```python
from build123d import *

# Parameters (mm, degrees)
SKETCH001_W  = 448.31
SKETCH001_H  = 304.8
PAD_DEPTH    = 4.318
POCKET_DEPTH = 1088.576426


with BuildPart() as part:
    # Sketch001 → Pad (new body)
    with BuildSketch(Plane.YZ):
        with Locations((0, 101.6)):
            Rectangle(SKETCH001_W, SKETCH001_H)
    extrude(amount=PAD_DEPTH)

    # Sketch (on Face6 of Pad) → Pocket (cut, through all)
    with BuildSketch(Plane.YZ.offset(4.318)):
        with BuildLine():
            ThreePointArc((-32.844781, 108.076032), (-32.844781, 135.0168), (-59.785549, 135.0168))
            Line((-59.785549, 135.0168), (-155.38703, 39.41532))
            ThreePointArc((-155.38703, 39.41532), (-155.38703, 12.474551), (-128.446262, 12.474551))
            Line((-32.844781, 108.076032), (-128.446262, 12.474551))
        make_face()
        with BuildLine():
            Line((-13.470384, 64.588636), (-56.59327, 21.46575))
            ThreePointArc((-56.59327, 21.46575), (-60.722791, 0.705246), (-43.122886, -11.054634))
            Line((-43.122886, -11.054634), (0, -11.054634))
            Line((0, 70.168252), (0, -11.054634))
            ThreePointArc((0, 70.168252), (-7.290119, 68.718157), (-13.470384, 64.588636))
        make_face()
        with BuildLine():
            Line((-183.066243, 203.2), (-100.454911, 203.2))
            ThreePointArc((-86.984527, 170.679616), (-82.855006, 191.440119), (-100.454911, 203.2))
            Line((-86.984527, 170.679616), (-159.575036, 98.089107))
            ThreePointArc((-192.09542, 111.559491), (-180.33554, 93.959586), (-159.575036, 98.089107))
            Line((-192.09542, 111.559491), (-192.09542, 194.170823))
            ThreePointArc((-183.066243, 203.2), (-189.450836, 200.555415), (-192.09542, 194.170823))
        make_face()
    pocket = extrude(amount=-POCKET_DEPTH, mode=Mode.SUBTRACT)

    # Mirrored: Pocket across Sketch V_Axis
    add(pocket.mirror(Plane(origin=(4.318, 0, 0), x_dir=(1, 0, 0), z_dir=(0, 1, 0))), mode=Mode.SUBTRACT)


solid = part.part
```
Geometry: final body of the model. Coordinates: model frame, mm. A direction names the side the tool comes from. Round coordinates to 2 decimals unless told otherwise and drop trailing zeros. Write each loop counter-clockwise with the first axis right and the second up, starting at its lowest first coordinate (ties: lowest second). Pieces come first, ordered by that corner, then holes.
Item 1: Section query D-D (y = 106). Return loops of the section in (x, z).
Item 2: Section query C-C (z = 150). Return loops of the section in (x, y) (3 decimals).
Item 3: Section query B-B (y = -169.5). Return loops of the section in (x, z), plus the area to 3 significant figures.
Item 4: Section query A-A (x = 1.2). Give the number of separate pieces and of enclosed holes in the cut face, plus the area to 4 significant figures.
Item 5: Material intervals for L1, parallel to Y at x = 3.75, z = 182.5 (1 decimal); L2, parallel to Z at x = 1.3, y = -135; L3, parallel to Y at x = 3.5, z = 193.5 (3 decimals), sorted ascending.
Item 6: Set-up query: faces 1 (the face through (0, -3, 104)), 2 (the face through (2.19, 180.62, 94.08)). Return all of +Z, -Z, +X, -X, +Y, -Y with unobstructed straight access to the full face (end or side cutting, diameter ignored); none if empty.
Completed:
1. outline: (0, -50.8) - (4.32, -50.8) - (4.32, 34.92) - (0, 34.92) - close; (0, 88.8) - (4.32, 88.8) - (4.32, 151.66) - (0, 151.66) - close; (0, 203.2) - (4.32, 203.2) - (4.32, 254) - (0, 254) - close
2. outline: (0, -224.155) - (4.318, -224.155) - (4.318, -192.095) - (0, -192.095) - close; (0, -107.664) - (4.318, -107.664) - (4.318, 107.664) - (0, 107.664) - close; (0, 192.095) - (4.318, 192.095) - (4.318, 224.155) - (0, 224.155) - close
3. outline: (0, -50.8) - (4.32, -50.8) - (4.32, 92.84) - (0, 92.84) - close; (0, 203.2) - (4.32, 203.2) - (4.32, 254) - (0, 254) - close
3. area: 840 mm2
4. separate pieces: 1
4. enclosed holes: 5
4. area: 100,000 mm2
5. L1: y = -224.2 to -192.1, -81.5 to 81.5, 192.1 to 224.2
5. L2: z = -50.8 to 8.19, 59.8 to 122.66, 203.2 to 254
5. L3: y = -224.155 to -192.095, -83.857 to 83.857, 192.095 to 224.155
6. face 1: +Z, -Z, -X, +Y, -Y
6. face 2: +X, -X
